For this review, take the finished solid that the model builds, in its own axes (mm). A direction names the side the tool comes from. Coordinates: 2 decimals unless noted, no trailing zeros. Write each loop counter-clockwise with the first axis right and the second up, starting at its lowest first coordinate (ties: lowest second). Pieces come first, ordered by that corner, then holes. Notation, with made-up numbers: (-28, 23.25) -> (11, 23.25) arc R4 cw to (11, 29.25) -> close; hole circle Ø9 at (5.5, 81). An arc over 180 degrees is marked (long way). One line per item, written item: value. Start each with the question number.
1) For pin 1 Ø2.5 at (y, z) = (4.5, 29) entering from -X; pin 2 Ø11 at (x, z) = (-3.5, 31.5) entering from +Y; pin 3 Ø2 at (y, z) = (6, 25.5) entering from +X; pin 4 Ø2.5 at (x, z) = (-20.5, -18) entering from -Y, all flat-tipped, find the tip position at first contact; note any pin that passes through.
2) Add section C-C (x = 9). State the section outline as (y, z) points, and give its area (3 significant figures).
3) Machinability: for faces 1 (the flat face through (0, 10.9, 17)), 2 (the flat face through (0, 7, -15.5)), 3 (the flat face through (19.61, 3, 29)), 4 (the flat face through (0, 5.9, 30)), 5 (the cylindrical face through (-18.914, 5.374, -18.208)), which of the approach directions +Z, -Z, +X, -X, +Y, -Y give a long, thin tool a straight path to every point of the face, cutting with its end or side? Answer none if there is none.
4) Add section A-A (y = 4.5). State the section outline as (x, z) points (3 decimals).
5) For probe 1 along X at (y, z) = (3.9, 30); probe 2 along X at (y, z) = (8, 18); probe 3 along X at (y, z) = (4, -1.5), list the stretches that pass through material, from the lowest coordinate up. Write a range as from..to.
6) Mouldability with a two-part tool opening along X and no side actions: class faces 6 (the flat face through (0, 5, -23)), 7 (the cylindrical face through (24, 5.53, -21.57)), 8 (the cylindrical face through (22.086, 5.374, 17.792)) as released by +X, released by -X, zero draft, split by the parting line, or undercut.
7) Add section B-B (y = 1.25). State the section outline as (x, z) points (3 decimals).
8) Add section D-D (z = 26). State the section outline as (x, y) points, and give its area (3 significant figures).
from build123d import *

# Parameters (mm, degrees)
SKETCH_1_W          = 51
SKETCH_1_H          = 46
SKETCH_1_R          = 1.6
SKETCH_1_W_2        = 39.22
SKETCH_1_H_2        = 12
EXTRUDE_1_DEPTH     = 10.9
SKETCH_2_W          = 39.22
SKETCH_2_H          = 10.3
CUT_EXTRUDE_1_DEPTH = 5
FILLET_1_R          = 5
SKETCH_3_W          = 36
SKETCH_3_H          = 31
CUT_EXTRUDE_2_DEPTH = 7.9
FILLET_3_R          = 4
FILLET_2_R          = 5


with BuildPart() as part:
    # ｽｹｯﾁ1 → ﾎﾞｽ - 押し出し1 (new body)
    # profile 1 of 2: a face of its own
    with BuildSketch(Plane(origin=(0, 0, 0), x_dir=(1, 0, 0), z_dir=(0, 1, 0))):
        Rectangle(SKETCH_1_W, SKETCH_1_H)
        with Locations(Location((-20.5, 18, 0), (0, 0, 270))):
            Circle(SKETCH_1_R, mode=Mode.SUBTRACT)
        with Locations(Location((20.5, 18, 0), (0, 0, 270))):
            Circle(SKETCH_1_R, mode=Mode.SUBTRACT)
        with Locations(Location((-20.5, -18, 0), (0, 0, 270))):
            Circle(SKETCH_1_R, mode=Mode.SUBTRACT)
        with Locations(Location((20.5, -18, 0), (0, 0, 270))):
            Circle(SKETCH_1_R, mode=Mode.SUBTRACT)
    # profile 2 of 2: a face of its own
    with BuildSketch(Plane(origin=(0, 0, 0), x_dir=(1, 0, 0), z_dir=(0, 1, 0))):
        with Locations((0, -29)):
            Rectangle(SKETCH_1_W_2, SKETCH_1_H_2)
        with Locations(Location((-14.61, -30, 0), (0, 0, 270))):
            Circle(SKETCH_1_R, mode=Mode.SUBTRACT)
        with Locations(Location((14.61, -30, 0), (0, 0, 270))):
            Circle(SKETCH_1_R, mode=Mode.SUBTRACT)
    extrude(amount=EXTRUDE_1_DEPTH)

    # ｽｹｯﾁ2 → ｶｯﾄ - 押し出し1 (cut)
    with BuildSketch(Plane(origin=(0, 10.9, 0), x_dir=(1, 0, 0), z_dir=(0, 1, 0))):
        with Locations((0, -30)):
            Rectangle(SKETCH_2_W, SKETCH_2_H)
    extrude(amount=-CUT_EXTRUDE_1_DEPTH, mode=Mode.SUBTRACT)

    # ﾌｨﾚｯﾄ1
    fillet_1_edges = [part.edges().sort_by_distance(p)[0] for p in [
        (-25.5, 5.45, 23),
        (-25.5, 5.45, -23),
        (25.5, 5.45, -23),
        (25.5, 5.45, 23),
        (19.61, 2.95, 35),
        (-19.61, 2.95, 35),
    ]]
    fillet(fillet_1_edges, radius=FILLET_1_R)

    # ｽｹｯﾁ3 → ｶｯﾄ - 押し出し2 (cut)
    with BuildSketch(Plane(origin=(0, 10.9, 0), x_dir=(1, 0, 0), z_dir=(0, 1, 0))):
        Rectangle(SKETCH_3_W, SKETCH_3_H)
    extrude(amount=-CUT_EXTRUDE_2_DEPTH, mode=Mode.SUBTRACT)

    # ﾌｨﾚｯﾄ3
    fillet_3_edges = [part.edges().sort_by_distance(p)[0] for p in [
        (18, 6.95, -15.5),
        (18, 6.95, 15.5),
        (-18, 6.95, 15.5),
        (-18, 6.95, -15.5),
    ]]
    fillet(fillet_3_edges, radius=FILLET_3_R)

    # ﾌｨﾚｯﾄ2
    # the kernel refuses this fillet: 5 mm, written as the material it adds along each edge
    with BuildSketch(Plane(origin=(-19.61, 0, 23), x_dir=(-0.9889327426199618, 0, -0.14836451925632577), z_dir=(0, 1, 0))) as fillet_2_piece_1_section:
        with BuildLine():
            CenterArc((4.333942914, 4.812619291), FILLET_2_R, 188.532159938, 65.732331269)
            Line((-0.610720799, 4.070796695), (-1.10518717, 3.996614435))
            Line((-1.10518717, 3.996614435), (-0.494466371, -0.07418226))
            Line((-0.494466371, -0.07418226), (0.07418226, -0.494466371))
            ThreePointArc((0.07418226, -0.494466371), (0.954332401, -0.362421949), (2.842359317, -0.481261929))
            Line((2.842359317, -0.481261929), (2.977957826, 0))
        make_face()
    fillet_2_piece_1 = extrude(amount=10.9, mode=Mode.PRIVATE)
    fillet_2_piece_1 = split(fillet_2_piece_1, bisect_by=Plane(origin=(-20.366453669, 5.9, 23.394752077), z_dir=(0, -1, 0)), keep=Keep.TOP, mode=Mode.PRIVATE)
    fillet_2_piece_1 = split(fillet_2_piece_1, bisect_by=Plane(origin=(-20.366453669, 2.95, 24.85), z_dir=(0, 0, -1)), keep=Keep.TOP, mode=Mode.PRIVATE)
    add(fillet_2_piece_1)
    with BuildSketch(Plane(origin=(-19.61, 0, 23), x_dir=(-0.9889327426199618, 0, -0.14836451925632577), z_dir=(0, 1, 0))) as fillet_2_piece_2_section:
        with BuildLine():
            CenterArc((4.333942914, 4.812619291), FILLET_2_R, 188.532159938, 65.732331269)
            Line((-0.610720799, 4.070796695), (-1.10518717, 3.996614435))
            Line((-1.10518717, 3.996614435), (-0.494466371, -0.07418226))
            Line((-0.494466371, -0.07418226), (0.07418226, -0.494466371))
            ThreePointArc((0.07418226, -0.494466371), (0.954332401, -0.362421949), (2.842359317, -0.481261929))
            Line((2.842359317, -0.481261929), (2.977957826, 0))
        make_face()
    fillet_2_piece_2 = extrude(amount=10.9, mode=Mode.PRIVATE)
    fillet_2_piece_2 = split(fillet_2_piece_2, bisect_by=Plane(origin=(-19.467497884, 5.9, 25.833436825), z_dir=(0, -1, 0)), keep=Keep.TOP, mode=Mode.PRIVATE)
    fillet_2_piece_2 = split(fillet_2_piece_2, bisect_by=Plane(origin=(-19.467497884, 2.95, 24.85), z_dir=(0, 0, 1)), keep=Keep.TOP, mode=Mode.PRIVATE)
    add(fillet_2_piece_2)
    with BuildSketch(Plane(origin=(-19.61, 0, 23), x_dir=(-0.9889327426199618, 0, -0.14836451925632577), z_dir=(0, 1, 0))) as fillet_2_piece_3_section:
        with BuildLine():
            CenterArc((4.333942914, 4.812619291), FILLET_2_R, 188.532159938, 65.732331269)
            Line((-0.610720799, 4.070796695), (-1.10518717, 3.996614435))
            Line((-1.10518717, 3.996614435), (-0.494466371, -0.07418226))
            Line((-0.494466371, -0.07418226), (0.07418226, -0.494466371))
            ThreePointArc((0.07418226, -0.494466371), (0.954332401, -0.362421949), (2.842359317, -0.481261929))
            Line((2.842359317, -0.481261929), (2.977957826, 0))
        make_face()
    fillet_2_piece_3 = extrude(amount=10.9, mode=Mode.PRIVATE)
    fillet_2_piece_3 = split(fillet_2_piece_3, bisect_by=Plane(origin=(-20.366453669, 5.9, 23.394752077), z_dir=(0, 1, 0)), keep=Keep.TOP, mode=Mode.PRIVATE)
    fillet_2_piece_3 = split(fillet_2_piece_3, bisect_by=Plane(origin=(-20.366453669, 8.4, 24.85), z_dir=(0, 0, -1)), keep=Keep.TOP, mode=Mode.PRIVATE)
    add(fillet_2_piece_3)
    with BuildSketch(Plane(origin=(19.61, 0, 23), x_dir=(0, 0, 1), z_dir=(0, 1, 0))) as fillet_2_piece_4_section:
        with BuildLine():
            CenterArc((4.116353438, 5), FILLET_2_R, 204.267668731, 65.732331269)
            Line((-0.441823281, 2.945), (-0.897640953, 2.7395))
            ThreePointArc((-0.897640953, 2.7395), (-0.5, 0.89), (-0.5, 0))
            Line((-0.5, 0), (0, -0.5))
            Line((0, -0.5), (4.116353438, -0.5))
            Line((4.116353438, -0.5), (4.116353438, 0))
        make_face()
    fillet_2_piece_4 = extrude(amount=10.9, mode=Mode.PRIVATE)
    fillet_2_piece_4 = split(fillet_2_piece_4, bisect_by=Plane(origin=(19.467497884, 2.95, 24.85), z_dir=(0, 0, 1)), keep=Keep.TOP, mode=Mode.PRIVATE)
    fillet_2_piece_4 = split(fillet_2_piece_4, bisect_by=Plane(origin=(19.467497884, 5.9, 25.833436825), z_dir=(0, -1, 0)), keep=Keep.TOP, mode=Mode.PRIVATE)
    add(fillet_2_piece_4)
    with BuildSketch(Plane(origin=(19.61, 0, 23), x_dir=(0, 0, 1), z_dir=(0, 1, 0))) as fillet_2_piece_5_section:
        with BuildLine():
            CenterArc((4.116353438, 5), FILLET_2_R, 204.267668731, 65.732331269)
            Line((-0.441823281, 2.945), (-0.897640953, 2.7395))
            ThreePointArc((-0.897640953, 2.7395), (-0.5, 0.89), (-0.5, 0))
            Line((-0.5, 0), (0, -0.5))
            Line((0, -0.5), (4.116353438, -0.5))
            Line((4.116353438, -0.5), (4.116353438, 0))
        make_face()
    fillet_2_piece_5 = extrude(amount=10.9, mode=Mode.PRIVATE)
    fillet_2_piece_5 = split(fillet_2_piece_5, bisect_by=Plane(origin=(20.366453669, 2.95, 24.85), z_dir=(0, 0, -1)), keep=Keep.TOP, mode=Mode.PRIVATE)
    fillet_2_piece_5 = split(fillet_2_piece_5, bisect_by=Plane(origin=(20.366453669, 5.9, 23.394752077), z_dir=(0, -1, 0)), keep=Keep.TOP, mode=Mode.PRIVATE)
    add(fillet_2_piece_5)
    with BuildSketch(Plane(origin=(19.61, 0, 23), x_dir=(0, 0, 1), z_dir=(0, 1, 0))) as fillet_2_piece_6_section:
        with BuildLine():
            CenterArc((4.116353438, 5), FILLET_2_R, 204.267668731, 65.732331269)
            Line((-0.441823281, 2.945), (-0.897640953, 2.7395))
            ThreePointArc((-0.897640953, 2.7395), (-0.5, 0.89), (-0.5, 0))
            Line((-0.5, 0), (0, -0.5))
            Line((0, -0.5), (4.116353438, -0.5))
            Line((4.116353438, -0.5), (4.116353438, 0))
        make_face()
    fillet_2_piece_6 = extrude(amount=10.9, mode=Mode.PRIVATE)
    fillet_2_piece_6 = split(fillet_2_piece_6, bisect_by=Plane(origin=(20.366453669, 8.4, 24.85), z_dir=(0, 0, -1)), keep=Keep.TOP, mode=Mode.PRIVATE)
    fillet_2_piece_6 = split(fillet_2_piece_6, bisect_by=Plane(origin=(20.366453669, 5.9, 23.394752077), z_dir=(0, 1, 0)), keep=Keep.TOP, mode=Mode.PRIVATE)
    add(fillet_2_piece_6)


solid = part.part
Numbers:
1. pin 1: x = -19.61
1. pin 2: y = 5.9
1. pin 3: x = 20.35
1. pin 4: through
2. outline: (0, -23) -> (10.9, -23) -> (10.9, -15.5) -> (3, -15.5) -> (3, 15.5) -> (10.9, 15.5) -> (10.9, 24.85) -> (5.9, 24.85) -> (5.9, 35) -> (0, 35) -> close
2. area: 337 mm²
3. face 1: +Z, -Z, +X, -X, +Y
3. face 2: +Y
3. face 3: +Z, +X, +Y, -Y
3. face 4: +Z, +X, -X, +Y
3. face 5: +Y, -Y
4. outline: (-25.5, -18) arc R5 ccw to (-20.5, -23) -> (20.5, -23) arc R5 ccw to (25.5, -18) -> (25.5, 18) arc R5 ccw to (22.555, 22.558) arc R5 cw to (19.61, 27.116) -> (19.61, 30) arc R5 ccw to (14.61, 35) -> (-14.61, 35) arc R5 ccw to (-19.61, 30) -> (-19.61, 27.116) arc R5 cw to (-22.555, 22.558) arc R5 ccw to (-25.5, 18) -> close; hole circle Ø3.2 at (-20.5, -18); hole circle Ø3.2 at (-20.5, 18); hole (-18, -11.5) arc R4 ccw to (-14, -15.5) -> (14, -15.5) arc R4 ccw to (18, -11.5) -> (18, 11.5) arc R4 ccw to (14, 15.5) -> (-14, 15.5) arc R4 ccw to (-18, 11.5) -> close; hole circle Ø3.2 at (-14.61, 30); hole circle Ø3.2 at (14.61, 30); hole circle Ø3.2 at (20.5, -18); hole circle Ø3.2 at (20.5, 18)
5. probe 1: -19.61..-16.21, -13.01..13.01, 16.21..19.61
5. probe 2: -25.5..-22.1, -18.9..18.9, 22.1..25.5
5. probe 3: -25.5..-18, 18..25.5
6. face 6: zero draft
6. face 7: released by +X
6. face 8: undercut
7. outline: (-25.5, -18) arc R5 ccw to (-20.5, -23) -> (20.5, -23) arc R5 ccw to (25.5, -18) -> (25.5, 18) arc R5 ccw to (22.555, 22.558) arc R5 cw to (19.61, 27.116) -> (19.61, 30) arc R5 ccw to (14.61, 35) -> (-14.61, 35) arc R5 ccw to (-19.61, 30) -> (-19.61, 27.116) arc R5 cw to (-22.555, 22.558) arc R5 ccw to (-25.5, 18) -> close; hole circle Ø3.2 at (-20.5, -18); hole circle Ø3.2 at (-20.5, 18); hole circle Ø3.2 at (-14.61, 30); hole circle Ø3.2 at (14.61, 30); hole circle Ø3.2 at (20.5, -18); hole circle Ø3.2 at (20.5, 18)
8. outline: (-19.74, 0) -> (19.74, 0) -> (19.74, 5.9) -> (-19.74, 5.9) -> close
8. area: 233 mm²
